Check sheet for the modelled part. Datum: model origin and axes. Units: mm. A direction names the side the tool comes from. Round coordinates to 2 decimals unless told otherwise and drop trailing zeros. Order: outer loops, then holes, each group sorted by start corner. A loop starts at its lowest first (then second) coordinate and runs counter-clockwise, first axis right, second up. Notation, with made-up numbers: (50, -17) -> (97, -17) arc R19 cw to (97, -6) -> close; hole circle Ø10 at (11, -32). An arc over 180 degrees is marked (long way). Use CSV: the item, a comma, the result in double quotes.
```python
from build123d import *

# Parameters (mm, degrees)
F1_DEPTH = 56
F2_R     = 1
F3_DEPTH = 1
F4_R     = 1
F5_DEPTH = 1


with BuildPart() as f1:
    # F0 (on Top) → F1 (new body)
    with BuildSketch(Plane.XY):
        Polygon((0, 9), (0, 0), (9, 0), (9, 1), (1, 1), (1, 9), align=None)
    extrude(amount=F1_DEPTH)

    # F2 (on face) → F3 (cut, through all)
    with BuildSketch(Plane.XZ):
        with Locations((5, 50.5)):
            Circle(F2_R)
        with Locations((5, 5.5)):
            Circle(F2_R)
    extrude(amount=-F3_DEPTH, mode=Mode.SUBTRACT)

    # F4 (on face) → F5 (cut, through all)
    with BuildSketch(Plane(origin=(0, 0, 0), x_dir=(0, -1, 0), z_dir=(-1, 0, 0))):
        with Locations((-5, 48)):
            Circle(F4_R)
        with Locations((-5, 8)):
            Circle(F4_R)
        with Locations((-5, 13)):
            Circle(F4_R)
        with Locations((-5, 43)):
            Circle(F4_R)
    extrude(amount=-F5_DEPTH, mode=Mode.SUBTRACT)


solid = f1.part
```
Q1. Access from +Z, -Z, +X, -X, +Y, -Y to the whole of each face (thin tool, end or side, straight path). Record for faces 1 (the face through (5, 1, 28)), 2 (the face through (0.49, 5.13, 8.99)).
Result sheet:
face 1,"+Z, -Z, +X, +Y"
face 2,"+X, -X"
Q2. Sectioned sample at A-A, the plane y = 5. Enter the section's corners in (x, z), then the cut area to 3 significant figures.
Result sheet:
outline,"(0, 0) -> (1, 0) -> (1, 7) -> (0, 7) -> close; (0, 9) -> (1, 9) -> (1, 12) -> (0, 12) -> close; (0, 14) -> (1, 14) -> (1, 42) -> (0, 42) -> close; (0, 44) -> (1, 44) -> (1, 47) -> (0, 47) -> close; (0, 49) -> (1, 49) -> (1, 56) -> (0, 56) -> close"
area,"48.0 mm^2"
Q3. Sectioned sample at C-C, the plane z = 5.5. Enter the section's corners in (x, y), then the cut area to 3 significant figures.
Result sheet:
outline,"(0, 0) -> (4, 0) -> (4, 1) -> (1, 1) -> (1, 9) -> (0, 9) -> close; (6, 0) -> (9, 0) -> (9, 1) -> (6, 1) -> close"
area,"15.0 mm^2"
Q4. Go/stop test with flat-tipped pins: pin 1 (2.5 mm diameter, centred on y = 5, z = 8, fed in from -X); pin 2 (3 mm diameter, centred on x = 5, z = 5.5, fed in from +Y); pin 3 (1.6 mm diameter, centred on y = 5, z = 43, fed in from -X); pin 4 (2.5 mm diameter, centred on y = 5, z = 13, fed in from +X). Record where each tip stops, or that it passes through.
Result sheet:
pin 1,"stops at x = 0"
pin 2,"stops at y = 1"
pin 3,"passes through"
pin 4,"stops at x = 1"
Q5. Sectioned sample at B-B, the plane x = 5. Enter the section's corners in (y, z).
Result sheet:
outline,"(0, 0) -> (1, 0) -> (1, 4.5) -> (0, 4.5) -> close; (0, 6.5) -> (1, 6.5) -> (1, 49.5) -> (0, 49.5) -> close; (0, 51.5) -> (1, 51.5) -> (1, 56) -> (0, 56) -> close"
Q6. Mould release check, pull along X, two halves, no side actions. Record for faces 3 (the face through (9, 0.5, 27.6)), 4 (the face through (4.87, 0.49, 51.49)), 5 (the face through (0.5, 9, 27.6)): pulls with the +X half, pulls with the -X half, needs draft (parallel to the pull), parting line crosses it, or undercut.
Result sheet:
face 3,"pulls with the +X half"
face 4,"undercut"
face 5,"needs draft"
Q7. Sectioned sample at D-D, the plane z = 36. Enter the section's corners in (x, y).
Result sheet:
outline,"(0, 0) -> (9, 0) -> (9, 1) -> (1, 1) -> (1, 9) -> (0, 9) -> close"
Q8. Scan lines: L1, parallel to Z at x = 5, y = 0.35; L2, parallel to Z at x = 0.7, y = 5; L3, parallel to Y at x = 6.25, z = 12.5. Record each from-to range of solid material in increasing order.
Result sheet:
L1,"z = 0 to 4.5, 6.5 to 49.5, 51.5 to 56"
L2,"z = 0 to 7, 9 to 12, 14 to 42, 44 to 47, 49 to 56"
L3,"y = 0 to 1"
